Part print with two shaded views. Sizes in mm from the minimum x, y, z corner. Round coordinates to 2 decimals unless told otherwise and drop trailing zeros. Order: outer loops, then holes, each group sorted by start corner. A loop starts at its lowest first (then second) coordinate and runs counter-clockwise, first axis right, second up. Notation, with made-up numbers: M 19,6 L 24,6 A23 cw 24,34 Z; hole C -22,20 d3. An arc over 180 degrees is marked long. One line per question, with ' | ' between items.
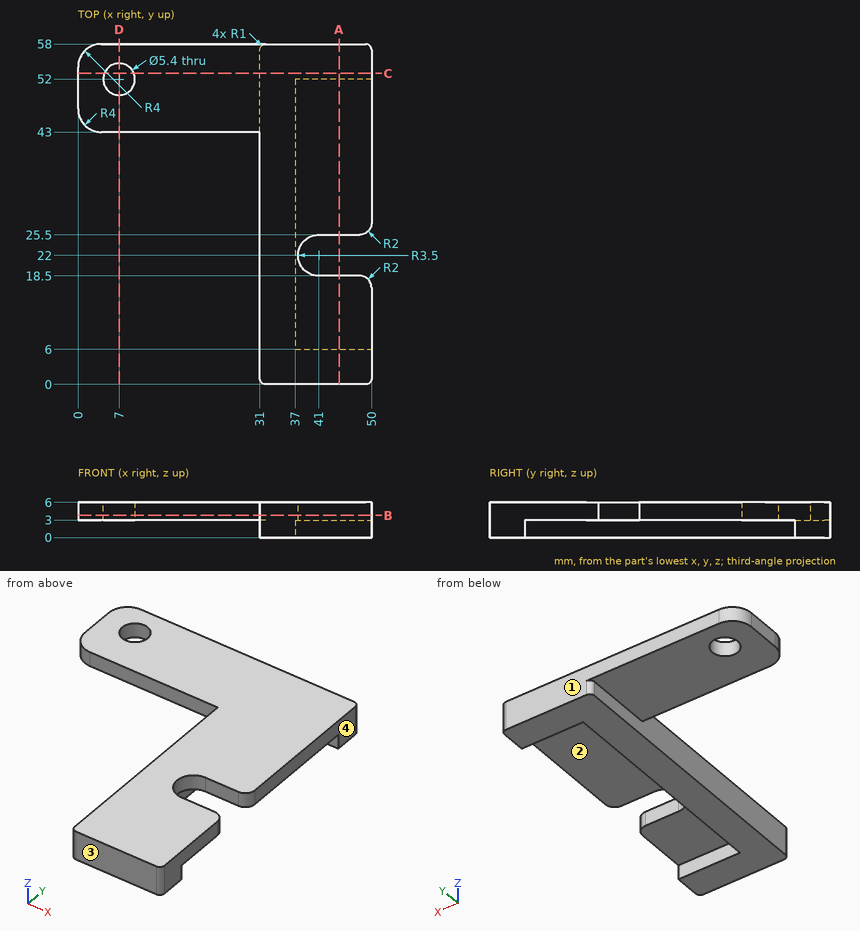
1) Saw through at B-B (z = 3.8). List the corners of the cut face in (x, y), plus the area to 3 significant figures.
The answers:
outline: M 0,47 A4 ccw 4,43 L 31,43 L 31,1 A1 ccw 32,0 L 49,0 A1 ccw 50,1 L 50,16.5 A2 ccw 48,18.5 L 41,18.5 A3.5 cw 41,25.5 L 48,25.5 A2 ccw 50,27.5 L 50,57 A1 ccw 49,58 L 4,58 A4 ccw 0,54 Z; hole C 7,52 d5.4 | area: 1,450 mm²
2) Probe line 1 (Y direction, x = 7, z = 3.8); line 2 (X direction, y = 35.5, z = 3.45); line 3 (Y direction, x = 13, z = 3.55). List the from-to ranges inside material, lowest first. Write a range as [from, to].
The answers:
line 1: y = [43, 49.3], [54.7, 58] | line 2: x = [31, 50] | line 3: y = [43, 58]
3) Two-plate mould, pull along Y, no slides. Class the marked faces 1, 2, 3 and 4: released by +Y, released by -Y, zero draft, split by the parting line, or undercut.
The answers:
face 1: released by +Y | face 2: undercut | face 3: released by -Y | face 4: zero draft
4) Saw through at D-D (x = 7). List the corners of the cut face in (y, z), plus the area to 3 significant figures.
The answers:
outline: M 43,3 L 49.3,3 L 49.3,6 L 43,6 Z; M 54.7,3 L 58,3 L 58,6 L 54.7,6 Z | area: 28.8 mm²
5) Drop flat-ended pins along their axis: pin 1 (7 mm diameter, centred on x = 7, y = 52, fed in from -Z); pin 2 (1.5 mm diameter, centred on x = 44, z = 4, fed in from -Y); pin 3 (2 mm diameter, centred on y = 44.5, z = 1.5, fed in from -X); pin 4 (2.5 mm diameter, centred on x = 17, z = 4.5, fed in from -Y). Give the stop position or say it passes through.
The answers:
pin 1: stops at z = 3 | pin 2: stops at y = 0 | pin 3: stops at x = 31 | pin 4: stops at y = 43
6) Saw through at C-C (y = 53). List the corners of the cut face in (x, z).
The answers:
outline: M 0,3 L 4.49,3 L 4.49,6 L 0,6 Z; M 9.51,3 L 31,3 L 31,0 L 50,0 L 50,6 L 9.51,6 Z
7) Saw through at A-A (x = 44.5). List the corners of the cut face in (y, z).
The answers:
outline: M 0,0 L 6,0 L 6,3 L 18.5,3 L 18.5,6 L 0,6 Z; M 25.5,3 L 52,3 L 52,0 L 58,0 L 58,6 L 25.5,6 Z
